```python
from build123d import *

# Parameters (mm, degrees)
CUT_EXTRUDE_1_REACH = 36.871
SKETCH_3_R          = 1.6
EXTRUDE_1_DEPTH     = 2
FILLET_1_R          = 3


with BuildPart() as part:
    # 草图1 → 旋转1 (revolve)
    with BuildSketch(Plane.XY, mode=Mode.PRIVATE) as revolve_1_sk:
        Polygon((0, 0), (21.320508076, 0), (24, 10), (21.929447639, 10), (19.7858541, 2), (0, 2), align=None)
    revolve(revolve_1_sk.sketch.rotate(Axis((0, 25.167510642, 0), (0, -1, 0)), 90), axis=Axis((0, 25.167510642, 0), (0, -1, 0)))

    # 草图2 → 切除-拉伸1 (cut, up to next)
    with BuildSketch(Plane(origin=(0, 2, 0), x_dir=(1, 0, 0), z_dir=(0, 1, 0)), mode=Mode.PRIVATE) as cut_extrude_1_sk1:
        with BuildLine():
            Line((11, 3), (0.32455532, 3))
            ThreePointArc((0.32455532, 3), (-13, 0), (0.32455532, -3))
            Line((0.32455532, -3), (11, -3))
            ThreePointArc((11, -3), (14, 0), (11, 3))
        make_face()
    cut_extrude_1_tool1 = extrude(cut_extrude_1_sk1.sketch, amount=-CUT_EXTRUDE_1_REACH, mode=Mode.PRIVATE) & part.part
    add(cut_extrude_1_tool1.solids().sort_by_distance((-1.696004, 2, 0))[0], mode=Mode.SUBTRACT)

    # 草图3 → 凸台-拉伸1 (add)
    # profile 1 of 2: a face of its own
    with BuildSketch(Plane(origin=(0, 10, 0), x_dir=(1, 0, 0), z_dir=(0, 1, 0))):
        with BuildLine():
            Line((-3.464101615, 14), (-7.316676114, 20.672854772))
            ThreePointArc((-7.316676114, 20.672854772), (0, 21.929447639), (7.316676114, 20.672854772))
            Line((7.316676114, 20.672854772), (3.464101615, 14))
            ThreePointArc((3.464101615, 14), (0, 12), (-3.464101615, 14))
        make_face()
        with Locations(Location((0, 16, 0), (0, 0, 270))):
            Circle(SKETCH_3_R, mode=Mode.SUBTRACT)
    # profile 2 of 2: a face of its own
    with BuildSketch(Plane(origin=(0, 10, 0), x_dir=(1, 0, 0), z_dir=(0, 1, 0))):
        with BuildLine():
            Line((3.464101615, -14), (7.316676114, -20.672854772))
            ThreePointArc((7.316676114, -20.672854772), (0, -21.929447639), (-7.316676114, -20.672854772))
            Line((-7.316676114, -20.672854772), (-3.464101615, -14))
            ThreePointArc((-3.464101615, -14), (0, -12), (3.464101615, -14))
        make_face()
        with Locations(Location((0, -16, 0), (0, 0, 90))):
            Circle(SKETCH_3_R, mode=Mode.SUBTRACT)
    extrude(amount=-EXTRUDE_1_DEPTH)

    # 圆角1
    fillet_1_edges = [part.edges().sort_by_distance(p)[0] for p in [
        (-7.180384511, 8.99998489, -20.436790791),
        (7.180384511, 8.99998489, -20.436790791),
        (-7.180384511, 8.99998489, 20.436790791),
        (7.180384511, 8.99998489, 20.436790791),
    ]]
    fillet(fillet_1_edges, radius=FILLET_1_R)


solid = part.part
```
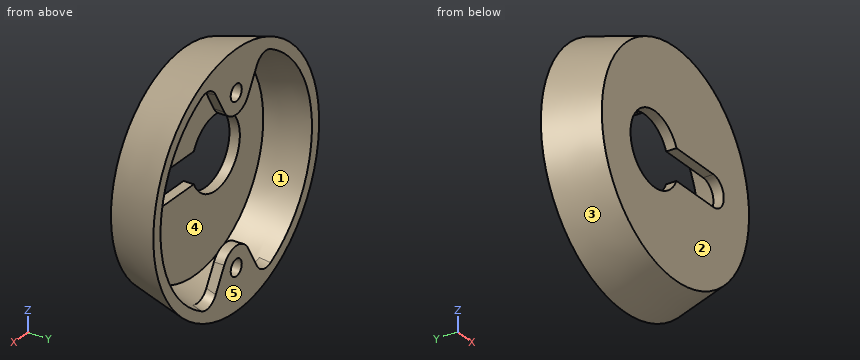
Work out the finished part from the listing and answer in its coordinate system (mm). Face numbers are marked on the shaded views. A direction names the side the tool comes from. Give positions to 0.01 mm unless a question says otherwise; leave off trailing zeros. Loops run counter-clockwise (first coordinate to the right, second up) from the corner with the lowest first, then second, coordinate; pieces in that order, holes last. Notation, with made-up numbers: (-3.75, -4) -> (13.25, -4) arc R24 ccw to (13.25, 27) -> close; hole circle Ø8 at (56.5, 9). An arc over 180 degrees is marked (long way). Put each result on its own line as item: value. Start each with the question number.
Item 1: Find the intervals of material crossed by L1, parallel to X at y = 9.55, z = 16; L2, parallel to X at y = 9, z = -16; L3, parallel to Z at x = 13.5, y = 6.75, in increasing order. Write a range as [from, to].
Item 2: Which of the six approach directions +Z, -Z, +X, -X, +Y, -Y give full straight-line access (tool end or side, diameter ignored) to the marked faces 4 and 5?
Item 3: The part is cut by section B-B (y = 7). Give the vertices of the cut face in (x, z).
Item 4: The mould has two halves that part along X. Classify the marked faces 1, 2 and 3: released by +X, released by -X, zero draft, split by the parting line, or undercut.
Item 5: The part is cut by section A-A (z = 0). Give the vertices of the cut face in (x, y).
Item 6: Each of these flat-tipped pins is pushed along its axis until it touches: P1, Ø3, axis at y = 2, z = -2, coming from the +X side; P2, Ø2, axis at x = 7, z = -8, coming from the +Y side; P3, Ø3, axis at y = 6, z = -6.5, coming from the +X side. Where does it stop, or does it pass through?
Answers below:
1. L1: [-17.73, -14.82], [-4.62, -1.6], [1.6, 4.62], [14.82, 17.73]
1. L2: [-17.53, -14.6], [-4.62, -1.6], [1.6, 4.62], [14.6, 17.53]
1. L3: [-18.78, -16.16], [16.16, 18.78]
2. face 4: none
2. face 5: +Z, -Z, +X, -X, +Y
3. outline: circle Ø46.39 at (0, 0); hole circle Ø42.25 at (0, 0)
4. face 1: undercut
4. face 2: zero draft
4. face 3: split by the parting line
5. outline: (-24, 10) -> (-21.32, 0) -> (-13, 0) -> (-13, 2) -> (-19.79, 2) -> (-21.93, 10) -> close; (14, 0) -> (21.32, 0) -> (24, 10) -> (21.93, 10) -> (19.79, 2) -> (14, 2) -> close
6. P1: x = 22.19
6. P2: y = 2
6. P3: x = 22.57
